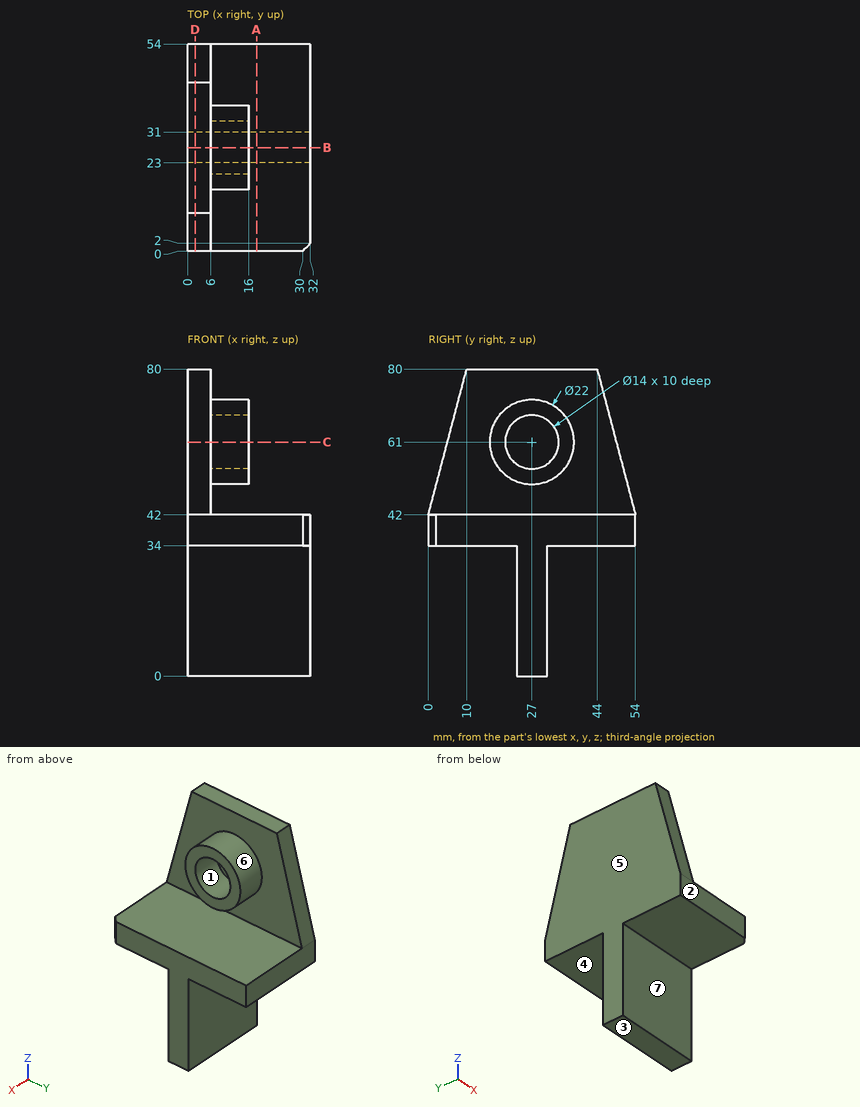
Geometry check sheet. Reference: drawing and pictorial views, mm from the part's lowest x, y, z. A direction names the side the tool comes from. Give positions to 0.01 mm unless a question says otherwise; leave off trailing zeros. Write each loop counter-clockwise with the first axis right and the second up, starting at its lowest first coordinate (ties: lowest second). Pieces come first, ordered by that corner, then holes. Notation, with made-up numbers: M 27.25,10.25 L 40.25,10.25 A14 cw 40.25,18.25 Z; hole C 23.5,42 d11. An arc over 180 degrees is marked long. Use CSV: the item, a comma, the result in double quotes.
1) Access from +Z, -Z, +X, -X, +Y, -Y to the whole of each face (thin tool, end or side, straight path). Record for the marked faces 4, 5, 6 and 7.
Final values:
face 4,"-Z, +X, -X, +Y"
face 5,"+Z, -Z, -X, +Y, -Y"
face 6,"+X"
face 7,"-Z, +X, -X, -Y"
2) Material ranges on line 1 along Z through (x, y) = (9, 27); line 2 along Z through (x, y) = (9.5, 8); line 3 along X through (y, z) = (33.5, 75.5), recorded low to high.
Final values:
line 1,"0 to 42, 50 to 54, 68 to 72"
line 2,"34 to 42"
line 3,"0 to 6"
3) Cross-section at C-C (z = 61). Enter the section's corners in (x, y), plus the area to 3 significant figures.
Final values:
outline,"M 0,5 L 6,5 L 6,16 L 16,16 L 16,20 L 6,20 L 6,34 L 16,34 L 16,38 L 6,38 L 6,49 L 0,49 Z"
area,"344 mm²"
4) Go/stop test with flat-tipped pins: pin 1 Ø7 at (x, y) = (18.5, 16) entering from -Z; pin 2 Ø11 at (y, z) = (26.5, 59.5) entering from +X; pin 3 Ø1.5 at (x, z) = (15, 19.5) entering from -Y. Record where each tip stops, or that it passes through.
Final values:
pin 1,"z = 34"
pin 2,"x = 16"
pin 3,"y = 23"
5) Cross-section at B-B (y = 27). Enter the section's corners in (x, z).
Final values:
outline,"M 0,0 L 32,0 L 32,42 L 6,42 L 6,50 L 16,50 L 16,54 L 6,54 L 6,68 L 16,68 L 16,72 L 6,72 L 6,80 L 0,80 Z"
6) Cross-section at A-A (x = 18). Enter the section's corners in (y, z), plus the area to 3 significant figures.
Final values:
outline,"M 0,34 L 23,34 L 23,0 L 31,0 L 31,34 L 54,34 L 54,42 L 0,42 Z"
area,"704 mm²"
7) Cross-section at D-D (x = 2). Enter the section's corners in (y, z), plus the area to 3 significant figures.
Final values:
outline,"M 0,34 L 23,34 L 23,0 L 31,0 L 31,34 L 54,34 L 54,42 L 44,80 L 10,80 L 0,42 Z"
area,"2,380 mm²"
8) Release check for a two-part mould opening along Z. For the marked faces 1, 2 and 3 record: released by +Z, released by -Z, zero draft, split by the parting line, or undercut.
Final values:
face 1,"undercut"
face 2,"zero draft"
face 3,"released by -Z"
